Check sheet for the modelled part. Datum: model origin and axes. Units: mm. Round coordinates to 2 decimals unless told otherwise and drop trailing zeros. Order: outer loops, then holes, each group sorted by start corner. A loop starts at its lowest first (then second) coordinate and runs counter-clockwise, first axis right, second up. Notation, with made-up numbers: M 88.5,-33.75 L 138.5,-33.75 A22 cw 138.5,2.25 Z; hole C -10.5,72 d11. An arc over 180 degrees is marked long. One line per item, written item: value. Start each with the question number.
(1) Cross-section at C-C, the plane x = 0. Enter the section's corners in (y, z), and give its area (3 significant figures).
(2) Cross-section at B-B, the plane y = 11.25. Enter the section's corners in (x, z).
(3) Release check for a two-part mould opening along Y. For faces 1 (the face through (12.14, -12.196, 7.213)), 2 (the face through (-12.14, 12.196, 7.213)), 3 (the face through (-8.73, 0.04, 7.21)) record: released by +Y, released by -Y, zero draft, split by the parting line, or undercut.
(4) Depth check by flat-ended pin: pin 1 Ø1 at (x, z) = (0, 13) entering from +Y; pin 2 Ø2 at (x, z) = (3, 10.5) entering from -Y; pin 3 Ø8 at (y, z) = (-1, 10.5) entering from -X. Enter the tip coordinate at first touch or a pass-through.
(5) Thickness scan on L1, parallel to X at y = -12, z = 10; L2, parallel to Y at x = -11.25, z = 3; L3, parallel to Y at x = 10.75, z = 2.5. Record the ranges inside material, lowest first.
(6) Cross-section at D-D, the plane y = -6.5. Enter the section's corners in (x, z), and give its area (3 significant figures).
(7) Cross-section at A-A, the plane x = 11. Enter the section's corners in (y, z), and give its area (3 significant figures).
from build123d import *

# Parameters (mm, degrees)
BOSS_EXTRUDE1_DEPTH = 14.63
FILLET1_START       = -1
FILLET1_DEPTH       = 17


with BuildPart() as part:
    # Sketch1 → Boss-Extrude1 (new body)
    with BuildSketch(Plane.XY):
        with BuildLine():
            Line((-8.519586833, 13.656293319), (-9.325754445, 14.46246093))
            ThreePointArc((-9.325754445, 14.46246093), (-12.168247041, 12.168247045), (-14.462460931, 9.325754452))
            Line((-14.462460931, 9.325754452), (-11.8745961, 6.737889618))
            Line((-11.874596103, 6.737889615), (-10.218772523, 5.082066036))
            Line((-10.218772523, 5.082066036), (-8.180331434, 3.043624946))
            ThreePointArc((-8.180331434, 3.043624946), (-8.7282, 0), (-8.18033144, -3.043624947))
            Line((-8.18033144, -3.043624947), (-10.218772531, -5.082066037))
            Line((-10.218772528, -5.082066035), (-13.656293332, -8.519586838))
            Line((-13.656293332, -8.519586838), (-14.462460943, -9.32575445))
            ThreePointArc((-14.462460943, -9.32575445), (-12.168247058, -12.168247046), (-9.325754465, -14.462460936))
            Line((-9.325754465, -14.462460936), (-8.519586857, -13.656293329))
            Line((-8.519586853, -13.656293332), (-5.082066058, -10.218772534))
            Line((-5.082066049, -10.218772528), (-3.043624959, -8.180331439))
            ThreePointArc((-3.043624959, -8.180331439), (-2.566843213, -8.342229394), (-2.081519018, -8.476364428))
            ThreePointArc((-2.081519021, -8.476364441), (-1e-08, -8.728200016), (2.081519001, -8.47636444))
            ThreePointArc((2.081518999, -8.476364431), (2.566843194, -8.342229397), (3.04362494, -8.180331443))
            Line((3.04362494, -8.180331443), (3.232471481, -8.369177985))
            Line((3.232471481, -8.369177985), (5.082066029, -10.218772535))
            Line((5.082066028, -10.21877254), (8.519586825, -13.656293337))
            Line((8.519586826, -13.656293336), (9.325754437, -14.462460949))
            ThreePointArc((9.325754437, -14.462460949), (12.168247033, -12.168247063), (14.462460923, -9.32575447))
            Line((14.462460923, -9.32575447), (13.656293316, -8.519586862))
            Line((13.656293316, -8.519586862), (10.218772514, -5.082066055))
            Line((10.218772514, -5.082066055), (8.180331425, -3.043624964))
            ThreePointArc((8.180331425, -3.043624964), (8.728199992, -1.8e-08), (8.180331432, 3.043624929))
            Line((8.180331432, 3.043624929), (10.218772523, 5.082066019))
            Line((10.218772523, 5.082066019), (13.656293323, 8.51958682))
            Line((13.656293323, 8.51958682), (14.462460935, 9.325754432))
            ThreePointArc((14.462460935, 9.325754432), (12.16824705, 12.168247028), (9.325754457, 14.462460918))
            Line((9.325754457, 14.462460918), (8.519586849, 13.65629331))
            Line((8.519586849, 13.65629331), (5.082066046, 10.218772512))
            Line((5.082066041, 10.21877251), (3.043624951, 8.18033142))
            ThreePointArc((3.043624951, 8.18033142), (5e-09, 8.728199987), (-3.043624942, 8.180331427))
            Line((-3.043624942, 8.180331427), (-3.232471485, 8.36917797))
            Line((-3.232471485, 8.36917797), (-5.082066032, 10.218772518))
            Line((-5.082066032, 10.218772518), (-8.519586833, 13.656293319))
        make_face()
    extrude(amount=BOSS_EXTRUDE1_DEPTH)

    # Fillet1: read off the stored shape, not the designer's step
    # Fillet1 outline → Fillet1 (cut)
    with BuildSketch(Plane.XY.offset(FILLET1_START)):
        with BuildLine():
            Line((14.462460923, -9.32575447), (13.877353973, -8.740647519))
            add(Edge.make_bspline(
                [(13.877353973, -8.740647519), (14.477597103, -9.34089065), (13.982799074, -10.030643172)],
                knots=[0, 0, 0, 1, 1, 1], degree=2, weights=[1, 0.76236352, 1]))
            ThreePointArc((13.982799074, -10.030643172), (14.226996208, -9.681169934), (14.462460923, -9.32575447))
        make_face()
        with BuildLine():
            ThreePointArc((9.325754437, -14.462460949), (9.681169902, -14.226996234), (10.03064314, -13.982799101))
            add(Edge.make_bspline(
                [(10.03064314, -13.982799101), (9.340890617, -14.477597129), (8.740647487, -13.877353998)],
                knots=[0, 0, 0, 1, 1, 1], degree=2, weights=[1, 0.76236352, 1]))
            Line((8.740647487, -13.877353998), (9.325754437, -14.462460949))
        make_face()
        with BuildLine():
            Line((-9.325754465, -14.462460936), (-8.740647514, -13.877353986))
            add(Edge.make_bspline(
                [(-8.740647514, -13.877353986), (-9.340890645, -14.477597116), (-10.030643167, -13.982799087)],
                knots=[0, 0, 0, 1, 1, 1], degree=2, weights=[1, 0.76236352, 1]))
            ThreePointArc((-10.030643167, -13.982799087), (-9.681169929, -14.226996221), (-9.325754465, -14.462460936))
        make_face()
        with BuildLine():
            ThreePointArc((-14.462460943, -9.32575445), (-14.226996229, -9.681169914), (-13.982799096, -10.030643153))
            add(Edge.make_bspline(
                [(-13.982799096, -10.030643153), (-14.477597124, -9.34089063), (-13.877353993, -8.7406475)],
                knots=[0, 0, 0, 1, 1, 1], degree=2, weights=[1, 0.76236352, 1]))
            Line((-13.877353993, -8.7406475), (-14.462460943, -9.32575445))
        make_face()
        with BuildLine():
            Line((-14.462460931, 9.325754452), (-13.877353981, 8.740647501))
            add(Edge.make_bspline(
                [(-13.877353981, 8.740647501), (-14.477597111, 9.340890632), (-13.982799082, 10.030643154)],
                knots=[0, 0, 0, 1, 1, 1], degree=2, weights=[1, 0.76236352, 1]))
            ThreePointArc((-13.982799082, 10.030643154), (-14.226996216, 9.681169916), (-14.462460931, 9.325754452))
        make_face()
        with BuildLine():
            ThreePointArc((-9.325754445, 14.46246093), (-9.681169909, 14.226996216), (-10.030643148, 13.982799083))
            add(Edge.make_bspline(
                [(-10.030643148, 13.982799083), (-9.340890625, 14.47759711), (-8.740647495, 13.87735398)],
                knots=[0, 0, 0, 1, 1, 1], degree=2, weights=[1, 0.76236352, 1]))
            Line((-8.740647495, 13.87735398), (-9.325754445, 14.46246093))
        make_face()
        with BuildLine():
            Line((9.325754457, 14.462460918), (8.740647501, 13.87735397))
            add(Edge.make_bspline(
                [(8.740647501, 13.87735397), (9.340890632, 14.477597101), (10.030643154, 13.982799072)],
                knots=[0, 0, 0, 1, 1, 1], degree=2, weights=[1, 0.76236352, 1]))
            ThreePointArc((10.030643154, 13.982799072), (9.681169919, 14.226996204), (9.325754457, 14.462460918))
        make_face()
        with BuildLine():
            ThreePointArc((14.462460935, 9.325754432), (14.226996221, 9.681169896), (13.982799088, 10.030643134))
            add(Edge.make_bspline(
                [(13.982799088, 10.030643134), (14.477597115, 9.340890612), (13.877353985, 8.740647482)],
                knots=[0, 0, 0, 1, 1, 1], degree=2, weights=[1, 0.76236352, 1]))
            Line((13.877353985, 8.740647482), (14.462460935, 9.325754432))
        make_face()
    extrude(amount=FILLET1_DEPTH, mode=Mode.SUBTRACT)


solid = part.part
Values found:
1. outline: M -8.73,0 L 8.73,0 L 8.73,14.63 L -8.73,14.63 Z
1. area: 255 mm^2
2. outline: M -13.02,0 L -6.11,0 L -6.11,14.63 L -13.02,14.63 Z; M 6.11,0 L 13.02,0 L 13.02,14.63 L 6.11,14.63 Z
3. face 1: released by -Y
3. face 2: released by +Y
3. face 3: undercut
4. pin 1: y = 8.73
4. pin 2: y = -9.14
4. pin 3: x = -10.14
5. L1: -12.33 to -6.86, 6.86 to 12.33
5. L2: -13.02 to -6.11, 6.11 to 13.02
5. L3: -13.44 to -5.61, 5.61 to 13.44
6. outline: M -11.64,0 L 11.64,0 L 11.64,14.63 L -11.64,14.63 Z
6. area: 340 mm^2
7. outline: M -13.23,0 L -5.86,0 L -5.86,14.63 L -13.23,14.63 Z; M 5.86,0 L 13.23,0 L 13.23,14.63 L 5.86,14.63 Z
7. area: 216 mm^2
